Autodesk Inventor part; units mm, degrees
ref_plane "YZ Plane" through (0, 0, 0) normal (1, 0, 0) x (0, 1, 0)
ref_plane "XZ Plane" through (0, 0, 0) normal (0, 1, 0) x (-1, 0, 0)
ref_plane "XY Plane" through (0, 0, 0) normal (0, 0, 1) x (1, 0, 0)
sketch "Sketch1" plane through (0, 0, 0) normal (0, 0, 1) x (1, 0, 0)
  line L0 (-22.6695, -7.62) -> (22.6695, -7.62)
  line L1 (22.6695, -7.62) -> (22.6695, 7.62)
  line L2 (22.6695, 7.62) -> (-22.6695, 7.62)
  line L3 (-22.6695, 7.62) -> (-22.6695, -7.62)
  line L4 (-22.6695, -7.62) -> (22.6695, 7.62) construction
  line L5 (22.6695, -7.62) -> (-22.6695, 7.62) construction
  point P0 (0, 0)
  dimension "d0" = 15.24
  dimension "d1" = 45.339
extrude "Extrusion1" add sketch "Sketch1" along normal blind 5.08
sketch "Sketch2" plane through (0, 0, 0) normal (0, 0, -1) x (-1, 0, 0)
  line L0 (22.6695, 7.62) -> (22.6695, -7.62)
  line L1 (-22.6695, -7.62) -> (-22.6695, 7.62)
  line L2 (-22.6695, 7.62) -> (22.6695, 7.62)
  point P0 (0, 0)
  point P1 (18.8595, 0)
  point P2 (-18.8595, 0)
  dimension "d4" = 3.81
  dimension "d5" = 3.81
  dimension "d6" = 7.62
  dimension "d7" = 7.62
  dimension "d35" = 15.24
hole "Hole1" at (-18.8595, 0, 0) at (18.8595, 0, 0) direction (0, 0, 1) diameter 3.175 end through all
sketch "Sketch3" plane through (0, 0, 0) normal (0, 0, -1) x (-1, 0, 0)
  circle A0 centre (0, 0) radius 1.524
  dimension "d15" = 3.048
extrude "Extrusion2" cut sketch "Sketch3" against normal through all
sketch "Sketch4" plane through (0, 0, 5.08) normal (0, 0, 1) x (1, 0, 0)
  line L0 (22.6695, 7.62) -> (-22.6695, 7.62)
  line L1 (-22.6695, -7.62) -> (22.6695, -7.62)
  line L2 (-3.81, 7.62) -> (-8.89, 7.62)
  line L3 (-8.89, 7.62) -> (-8.89, -7.62)
  line L4 (-8.89, -7.62) -> (-3.81, -7.62)
  line L5 (-3.81, -7.62) -> (-3.81, 7.62)
  line L6 (3.81, 7.62) -> (8.89, 7.62)
  line L7 (8.89, 7.62) -> (8.89, -7.62)
  line L8 (8.89, -7.62) -> (3.81, -7.62)
  line L9 (3.81, -7.62) -> (3.81, 7.62)
  point P0 (0, 0)
  dimension "d18" = 5.08
  dimension "d19" = 3.81
  dimension "d20" = 3.81
  dimension "d21" = 5.08
extrude "Extrusion3" add sketch "Sketch4" along normal blind 12.7 contours L7 L1 L9 L0 | L5 L1 L3 L0
sketch "Sketch5" plane through (-8.89, -7.62, 5.08) normal (-1, 0, 0) x (0, 0, 1)
  line L0 (12.7, 15.24) -> (12.7, 0)
  line L1 (0, 15.24) -> (12.7, 15.24)
  point P0 (-5.08, 7.62)
  point P1 (6.35, 7.62)
  dimension "d24" = 6.35
  dimension "d25" = 7.62
  dimension "d36" = 15.24
hole "Hole2" at (-8.89, 0, 11.43) direction (1, 0, 0) diameter 5.08 end through all
fillet "Fillet1" radius 3.175 2 edges at (-8.89, 0, 5.08) (8.89, 0, 5.08)
properties part number "LowerSpringMountFrontV2"
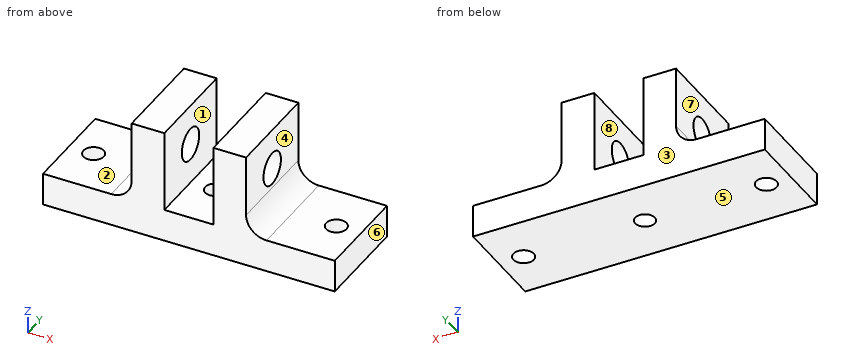
Geometry check sheet. Reference: the model listing, model coordinates, mm. Face numbers are marked on the shaded views. A direction names the side the tool comes from. Coordinates: 2 decimals unless noted, no trailing zeros. Order: outer loops, then holes, each group sorted by start corner. A loop starts at its lowest first (then second) coordinate and runs counter-clockwise, first axis right, second up.
Item 1: Section check D-D (x = 0). Enter the section's corners in (y, z), plus the area to 3 significant figures.
Item 2: Section check A-A (z = 11.43). Enter the section's corners in (x, y).
Item 3: Depth check by flat-ended pin: pin 1 (6 mm diameter, centred on x = 0.5, y = -3, fed in from +Z); pin 2 (8 mm diameter, centred on y = 0, z = 11.43, fed in from +X); pin 3 (5 mm diameter, centred on y = -2.5, z = 14.5, fed in from -X). Enter the tip coordinate at first touch or a pass-through.
Item 4: Tool access check on the marked faces 1, 2, 3 and 4. Record the directions out of +Z, -Z, +X, -X, +Y, -Y that give a thin tool (end or side, any length) a straight path to the whole face; none if there is none.
Item 5: Scan lines: line 1 along Z through (x, y) = (-5.95, 0); line 2 along Y through (x, z) = (-7.05, 11.43); line 3 along X through (y, z) = (4.5, 9.25). Record each from-to range of solid material in increasing order.
Item 6: Section check C-C (z = 14.75). Enter the section's corners in (x, y).
Item 7: Section check B-B (y = 0). Count the separate pieces of the cut face and the enclosed holes in it, plus the area to 3 significant figures.
Item 8: Mould release check, pull along X, two halves, no side actions. Record for the marked faces 5, 6, 7 and 8: released by +X, released by -X, zero draft, split by the parting line, or undercut.
Check sheet entries:
1. outline: (-7.62, 0) - (-1.52, 0) - (-1.52, 5.08) - (-7.62, 5.08) - close; (1.52, 0) - (7.62, 0) - (7.62, 5.08) - (1.52, 5.08) - close
1. area: 61.9 mm2
2. outline: (-8.89, -7.62) - (-3.81, -7.62) - (-3.81, -2.54) - (-8.89, -2.54) - close; (-8.89, 2.54) - (-3.81, 2.54) - (-3.81, 7.62) - (-8.89, 7.62) - close; (3.81, -7.62) - (8.89, -7.62) - (8.89, -2.54) - (3.81, -2.54) - close; (3.81, 2.54) - (8.89, 2.54) - (8.89, 7.62) - (3.81, 7.62) - close
3. pin 1: stops at z = 5.08
3. pin 2: stops at x = 9
3. pin 3: stops at x = -8.89
4. face 1: +Z, +Y, -Y
4. face 2: +Z, -X, +Y, -Y
4. face 3: +Z, -Z, +X, -X, +Y
4. face 4: +Z, +X, +Y, -Y
5. line 1: z = 0 to 8.89, 13.97 to 17.78
5. line 2: y = -7.62 to -2.54, 2.54 to 7.62
5. line 3: x = -8.89 to -3.81, 3.81 to 8.89
6. outline: (-8.89, -7.62) - (-3.81, -7.62) - (-3.81, 7.62) - (-8.89, 7.62) - close; (3.81, -7.62) - (8.89, -7.62) - (8.89, 7.62) - (3.81, 7.62) - close
7. separate pieces: 6
7. enclosed holes: 0
7. area: 264 mm2
8. face 5: zero draft
8. face 6: released by +X
8. face 7: released by -X
8. face 8: undercut
